Read the model definition and answer for the solid it produces. Units are mm, in the model's axes. Coordinates: 2 decimals unless noted, no trailing zeros. Order: outer loops, then holes, each group sorted by start corner. A loop starts at its lowest first (then second) coordinate and runs counter-clockwise, first axis right, second up. Notation, with made-up numbers: M -7,1 L 51,1 A11 ccw 51,13 Z; hole C 77.5,54 d2. An arc over 180 degrees is marked long. Use a Markdown table: item, result. Add a question column.
1) Each of these flat-tipped pins is pushed along its axis until it touches: pin 1 Ø1.2 at (y, z) = (0, 0) entering from -X; pin 2 Ø1.6 at (y, z) = (-0.5, 0) entering from -X; pin 3 Ø6 at (x, z) = (4, 13) entering from -Y. Where does it stop, or does it pass through?
2) Find section C-C on z = 15. Write down the section's boundary in (x, y), plus the area to 3 significant figures.
3) Find section D-D on x = 4. Write down the section's boundary in (y, z).
4) Find section B-B on y = 0. Write down the section's boundary in (x, z), plus the area to 3 significant figures.
5) Find the intervals of material crossed by probe 1 along Y at (x, z) = (-2.9, 0); probe 2 along Z at (x, y) = (-2.15, 0); probe 3 along Y at (x, z) = (-2.1, 0), in increasing order. Write a range as [from, to].
6) Find section A-A on x = -4. Write down the section's boundary in (y, z).
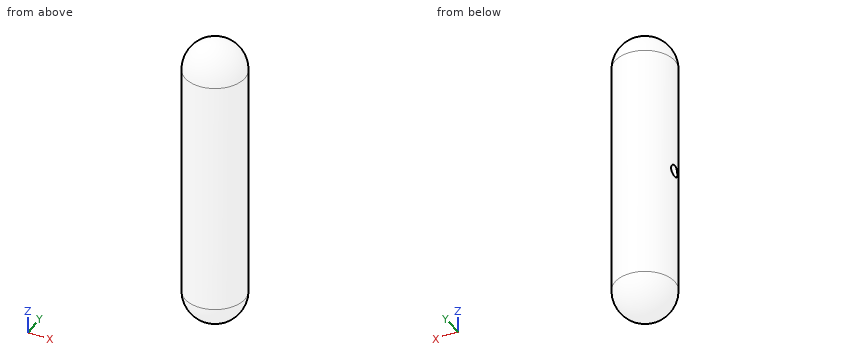
Solid Edge part; units mm, degrees
sketch "Sketch1" plane through (0, 0, 0) normal (1, 0, 0) x (0, 1, 0)
  line L0 (5, 25) -> (5, -25)
  line L1 (5, -25) -> (0, -25)
  line L2 (0, -25) -> (0, 0)
  line L3 (0, 0) -> (0, 25)
  line L4 (0, 25) -> (5, 25)
revolve "RevolvedProtrusion1" add sketch "Sketch1" angle 360 about axis through (0, 0, 0) along (0, 0, 1)
fillet "Round1" radius 5 2 edges at (-5, 0, 25) (-5, 0, -25)
hole "Hole_1" at (0, 0, 0) direction (-1, 0, 0) diameter 2 end up to next
properties material "Stainless steel"
Check result:
| question | item | result |
|---|---|---|
| 1 | pin 1 | stops at x = 0 |
| 1 | pin 2 | stops at x = -4.96 |
| 1 | pin 3 | stops at y = -4.9 |
| 2 | outline | C 0,0 d10 |
| 2 | area | 78.5 mm2 |
| 3 | outline | M -3,-20 A3 ccw 3,-20 L 3,20 A3 ccw -3,20 Z |
| 4 | outline | M -5,-20 A5 ccw 5,-20 L 5,20 A5 ccw -5,20 L -5,1 L 0,1 L 0,-1 L -5,-1 Z |
| 4 | area | 469 mm2 |
| 5 | probe 1 | y = [-4.07, -1], [1, 4.07] |
| 5 | probe 2 | z = [-24.51, -1], [1, 24.51] |
| 5 | probe 3 | y = [-4.54, -1], [1, 4.54] |
| 6 | outline | M -3,-20 A3 ccw 3,-20 L 3,20 A3 ccw -3,20 Z; hole C 0,0 d2 |
